```python
from build123d import *

# Parameters (mm, degrees)
SKETCH_1_W          = 10
SKETCH_1_H          = 10
EXTRUDE_1_DEPTH     = 4.4
SKETCH_2_W          = 12.4
SKETCH_2_H          = 12.4
EXTRUDE_2_DEPTH     = 3
SKETCH_3_R          = 1.8
CUT_EXTRUDE_1_DEPTH = 3
FILLET_1_R          = 1.2
CHAMFER_1_SIZE      = 0.4
CHAMFER_2_SIZE      = 0.4


with BuildPart() as part:
    # Эскиз1 → Бобышка-Вытянуть1 (new body)
    with BuildSketch(Plane.XY):
        with Locations((5, -5)):
            Rectangle(SKETCH_1_W, SKETCH_1_H)
    extrude(amount=EXTRUDE_1_DEPTH)

    # Эскиз2 → Бобышка-Вытянуть2 (add)
    with BuildSketch(Plane(origin=(0, 0, 0), x_dir=(-1, 0, 0), z_dir=(0, 0, -1))):
        with Locations((-5, -5)):
            Rectangle(SKETCH_2_W, SKETCH_2_H)
    extrude(amount=EXTRUDE_2_DEPTH)

    # Эскиз3 → Вырез-Вытянуть1 (cut)
    with BuildSketch(Plane(origin=(0, 0, -3), x_dir=(-1, 0, 0), z_dir=(0, 0, -1))):
        with Locations((-5, -5)):
            Circle(SKETCH_3_R)
    extrude(amount=-CUT_EXTRUDE_1_DEPTH, mode=Mode.SUBTRACT)

    # Скругление1
    fillet_1_edges = [part.edges().sort_by_distance(p)[0] for p in [
        (0, 0, 2.2),
        (10, 0, 2.2),
        (10, -10, 2.2),
        (0, -10, 2.2),
    ]]
    fillet(fillet_1_edges, radius=FILLET_1_R)

    # Фаска1
    chamfer_1_edges = [part.edges().sort_by_distance(p)[0] for p in [
        (5, 0, 4.4),
        (10, -5, 4.4),
        (0, -5, 4.4),
        (5, -10, 4.4),
        (9.648528137, -9.648528137, 4.4),
        (0.351471863, -9.648528137, 4.4),
        (0.351471863, -0.351471863, 4.4),
        (9.648528137, -0.351471863, 4.4),
    ]]
    chamfer(chamfer_1_edges, length=CHAMFER_1_SIZE)

    # Фаска2
    chamfer_2_edges = [part.edges().sort_by_distance(p)[0] for p in [
        (6.8, -5, -3),
    ]]
    chamfer(chamfer_2_edges, length=CHAMFER_2_SIZE)


solid = part.part
```
Can you work these out from the model? Positions are in its coordinate system, mm. A direction names the side the tool comes from. Coordinates: 2 decimals unless noted, no trailing zeros. Order: outer loops, then holes, each group sorted by start corner. A loop starts at its lowest first (then second) coordinate and runs counter-clockwise, first axis right, second up.
1. I'm going to push flat-ended pins straight in: pin 1 (1.1 mm diameter, centred on x = 5, y = -4.5, fed in from -Z); pin 2 (2 mm diameter, centred on y = -5, z = 1.5, fed in from +X). Where does each tip first touch, or does it pass through?
2. If we section it at A-A (z = -0.25): Please give me the cut outline in (x, y).
3. For faces 4 (the face through (0.342, -0.361, 2.028)), 5 (the face through (0, -5, 2)), 6 (the face through (10, -5, 2)), 7 (the face through (9.658, -9.639, 2.028)), 8 (the face through (5, -10, 2)), which set-ups out of +Z, -Z, +X, -X, +Y, -Y let a thin tool reach every point of the face, with its end or its side?
4. I need wall thicknesses on line 1 (Y direction, x = 5, z = -1.95); line 2 (Y direction, x = 6, z = 2.5); line 3 (Z direction, x = 10.25, y = 0.75). Which ranges of each line are inside material? Lowest first, please.
5. Thinking about a two-plate mould opening in X: for faces 1 (the face through (11.2, -5, -1)), 2 (the face through (0.534, -9.481, 4.247)), 3 (the face through (5, -5, 0)), which applies, +X half, -X half, draft (parallel to the pull), parting line (faces both ways), or undercut?
6. If we section it at D-D (z = 2): Please give me the cut outline in (x, y).
7. If we section it at C-C (x = 5): Please give me the cut outline in (y, z), then the cut area to 3 significant figures.
8. If we section it at B-B (y = -5): Please give me the cut outline in (x, z), then the cut area to 3 significant figures.
Entries:
1. pin 1: stops at z = 0
1. pin 2: stops at x = 10
2. outline: (-1.2, -11.2) - (11.2, -11.2) - (11.2, 1.2) - (-1.2, 1.2) - close; hole circle Ø3.6 at (5, -5)
3. face 4: +Z, -X, +Y
3. face 5: +Z, -X, +Y, -Y
3. face 6: +Z, +X, +Y, -Y
3. face 7: +Z, +X, -Y
3. face 8: +Z, +X, -X, -Y
4. line 1: y = -11.2 to -6.8, -3.2 to 1.2
4. line 2: y = -10 to 0
4. line 3: z = -3 to 0
5. face 1: +X half
5. face 2: -X half
5. face 3: undercut
6. outline: (0, -8.8) arc R1.2 ccw to (1.2, -10) - (8.8, -10) arc R1.2 ccw to (10, -8.8) - (10, -1.2) arc R1.2 ccw to (8.8, 0) - (1.2, 0) arc R1.2 ccw to (0, -1.2) - close
7. outline: (-11.2, -3) - (-7.2, -3) - (-6.8, -2.6) - (-6.8, 0) - (-3.2, 0) - (-3.2, -2.6) - (-2.8, -3) - (1.2, -3) - (1.2, 0) - (0, 0) - (0, 4) - (-0.4, 4.4) - (-9.6, 4.4) - (-10, 4) - (-10, 0) - (-11.2, 0) - close
7. area: 70.1 mm2
8. outline: (-1.2, -3) - (2.8, -3) - (3.2, -2.6) - (3.2, 0) - (6.8, 0) - (6.8, -2.6) - (7.2, -3) - (11.2, -3) - (11.2, 0) - (10, 0) - (10, 4) - (9.6, 4.4) - (0.4, 4.4) - (0, 4) - (0, 0) - (-1.2, 0) - close
8. area: 70.1 mm2
